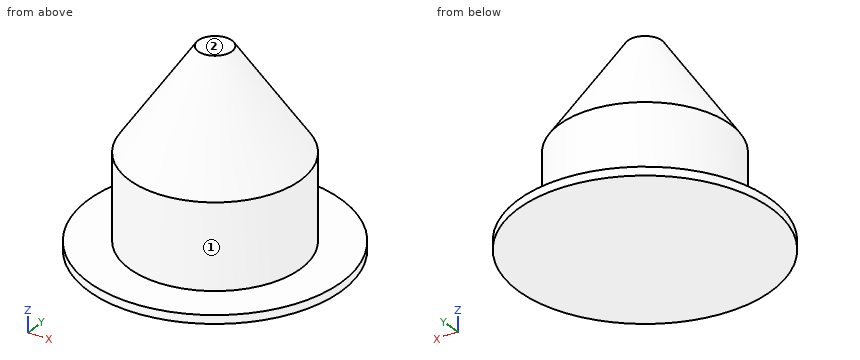
```python
from build123d import *

# Parameters (mm, degrees)
F0_R     = 19.05
F1_DEPTH = 1.27
F2_R     = 12.8905
F3_DEPTH = 12.7


with BuildPart() as f1:
    # F0 (on Top) → F1 (new body)
    with BuildSketch(Plane.XY):
        Circle(F0_R)
    extrude(amount=F1_DEPTH)

    # F2 (on face) → F3 (join)
    with BuildSketch(Plane.XY.offset(1.27)):
        Circle(F2_R)
    extrude(amount=F3_DEPTH)

    # F4 (on Front) → F5 (revolve)
    with BuildSketch(Plane.XZ):
        Polygon((2.54, 29.21), (0, 29.21), (0, 13.97), (12.8905, 13.97), align=None)
    revolve(axis=Axis((0, 0, 1.27), (0, 0, -1)))


solid = f1.part
```
For this review, take the finished solid that the model builds, in its own axes (mm). Face numbers are marked on the shaded views. A direction names the side the tool comes from. Give positions to 0.01 mm unless a question says otherwise; leave off trailing zeros. Loops run counter-clockwise (first coordinate to the right, second up) from the corner with the lowest first, then second, coordinate; pieces in that order, holes last. Notation, with made-up numbers: M -34,39.5 L 22,39.5 A30 cw 22,72.5 Z; hole C -17.75,84.25 d1. An arc over 180 degrees is marked long. One line per item, written item: value. Start each with the question number.
Q1. Clearance check with flat-ended pins moving along their axes: pin 1 Ø10 at (x, z) = (-4.5, 20.5) entering from -Y; pin 2 Ø1.5 at (x, z) = (10.5, 17) entering from -Y; pin 3 Ø1.5 at (x, y) = (0.5, 12) entering from +Z. State where each tip first meets the part, or that it passes through.
Q2. Machinability: for the marked faces 1 and 2, which of the approach directions +Z, -Z, +X, -X, +Y, -Y give a long, thin tool a straight path to every point of the face, cutting with its end or side? Answer none if there is none.
Q3. Add section D-D (z = 19.5). Give the boundary of the cut face in (x, y).
Q4. For L1, parallel to Z at x = -12.5, y = -8.5; L2, parallel to X at y = -1.5, z = 9.25; L3, parallel to Y at x = 5, z = 10, list the stretches that pass through material, from the lowest coordinate up.
Q5. Add section C-C (z = 8). Give the boundary of the cut face in (x, y).
Q6. Add section A-A (x = 0). Give the boundary of the cut face in (y, z).
Reply:
1. pin 1: y = -11.31
1. pin 2: y = -5.1
1. pin 3: z = 16.37
2. face 1: +Z
2. face 2: +Z, +X, -X, +Y, -Y
3. outline: C 0,0 d18.27
4. L1: 0 to 1.27
4. L2: -12.8 to 12.8
4. L3: -11.88 to 11.88
5. outline: C 0,0 d25.78
6. outline: M -19.05,0 L 19.05,0 L 19.05,1.27 L 12.89,1.27 L 12.89,13.97 L 2.54,29.21 L -2.54,29.21 L -12.89,13.97 L -12.89,1.27 L -19.05,1.27 Z
